from build123d import *

# Parameters (mm, degrees)
SKETCH1_W           = 136.32
SKETCH1_H           = 20
SKETCH1_R           = 5
BOSS_EXTRUDE1_DEPTH = 20
SKETCH2_R           = 2
CUT_EXTRUDE1_DEPTH  = 7.5
CUT_EXTRUDE2_START  = -7.5
SKETCH3_R           = 2
CUT_EXTRUDE2_DEPTH  = 7.5


with BuildPart() as part:
    # Sketch1 → Boss-Extrude1 (new body)
    with BuildSketch(Plane.XY):
        with Locations((68.16, 10)):
            Rectangle(SKETCH1_W, SKETCH1_H)
        with Locations((116.32, 10)):
            Circle(SKETCH1_R, mode=Mode.SUBTRACT)
        with Locations((20, 10)):
            Circle(SKETCH1_R, mode=Mode.SUBTRACT)
    extrude(amount=BOSS_EXTRUDE1_DEPTH)

    # Sketch2 → Cut-Extrude1 (cut)
    with BuildSketch(Plane.ZY):
        with Locations((10, 10)):
            Circle(SKETCH2_R)
    extrude(amount=-CUT_EXTRUDE1_DEPTH, mode=Mode.SUBTRACT)

    # Sketch3 → Cut-Extrude2 (cut)
    with BuildSketch(Plane(origin=(136.32, 0, 0), x_dir=(0, 0, -1), z_dir=(1, 0, 0)).offset(CUT_EXTRUDE2_START)):
        with Locations(Location((-10, 10, 0), (0, 0, 180))):
            Circle(SKETCH3_R)
    extrude(amount=CUT_EXTRUDE2_DEPTH, mode=Mode.SUBTRACT)


solid = part.part
Part model, mm, in its own coordinate system. A direction names the side the tool comes from. Coordinates: 2 decimals unless noted, no trailing zeros. Write each loop counter-clockwise with the first axis right and the second up, starting at its lowest first coordinate (ties: lowest second). Pieces come first, ordered by that corner, then holes. Notation, with made-up numbers: M 41,-39.75 L 96,-39.75 A18 ccw 96,-5.75 Z; hole C 70.5,80.5 d5. An arc over 180 degrees is marked long. Return JSON: item names as keys, results as strings.
1. 3-axis set-ups, long thin cutter, end or side, ignore diameter. For faces 4 (the face through (4, 12, 10)), 5 (the face through (67, 0, 10)), 6 (the face through (128.82, 10, 10)): which of +Z, -Z, +X, -X, +Y, -Y reach the whole face in a straight line?
Determined:
{"face 4": "-X", "face 5": "+Z, -Z, +X, -X, -Y", "face 6": "+X"}
2. Saw through at A-A, the plane x = 20. Write the cut outline in (y, z).
Determined:
{"outline": "M 0,0 L 5,0 L 5,20 L 0,20 Z; M 15,0 L 20,0 L 20,20 L 15,20 Z"}
3. Probe L1, parallel to Y at x = 20, z = 6; L2, parallel to Y at x = 131.25, z = 10. List the from-to ranges inside material, lowest first.
Determined:
{"L1": "0 to 5, 15 to 20", "L2": "0 to 8, 12 to 20"}
4. Saw through at D-D, the plane z = 16.25. Write the cut outline in (x, y).
Determined:
{"outline": "M 0,0 L 136.32,0 L 136.32,20 L 0,20 Z; hole C 20,10 d10; hole C 116.32,10 d10"}
5. Pull direction X, two halves, no side cores. Call faces 1 (the face through (0, 9.9, 7.6)), 2 (the face through (67, 20, 10)), 3 (the face through (19.349, 14.957, 9.86)): pulls with the +X half, pulls with the -X half, needs draft (parallel to the pull), parting line crosses it, or undercut.
Determined:
{"face 1": "pulls with the -X half", "face 2": "needs draft", "face 3": "undercut"}
6. Flat gauge pins, fed straight in: pin 1 Ø1.2 at (y, z) = (11, 10) entering from -X; pin 2 Ø3 at (y, z) = (10, 10) entering from +X. Where does each tip first touch, or does it go through?
Determined:
{"pin 1": "x = 7.5", "pin 2": "x = 128.82"}
7. Saw through at B-B, the plane z = 10. Write the cut outline in (x, y).
Determined:
{"outline": "M 0,0 L 136.32,0 L 136.32,8 L 128.82,8 L 128.82,12 L 136.32,12 L 136.32,20 L 0,20 L 0,12 L 7.5,12 L 7.5,8 L 0,8 Z; hole C 20,10 d10; hole C 116.32,10 d10"}
8. Saw through at C-C, the plane y = 10. Write the cut outline in (x, z), then the cut area to 3 significant figures.
Determined:
{"outline": "M 0,0 L 15,0 L 15,20 L 0,20 L 0,12 L 7.5,12 L 7.5,8 L 0,8 Z; M 25,0 L 111.32,0 L 111.32,20 L 25,20 Z; M 121.32,0 L 136.32,0 L 136.32,8 L 128.82,8 L 128.82,12 L 136.32,12 L 136.32,20 L 121.32,20 Z", "area": "2,270 mm²"}
